Source: CAD feature listing. Evaluate the final solid. Frame: model axes, mm. A direction names the side the tool comes from. Give positions to 0.01 mm unless a question says otherwise; leave off trailing zeros. Order: outer loops, then holes, each group sorted by start corner. A loop starts at its lowest first (then second) coordinate and runs counter-clockwise, first axis right, second up. Notation, with made-up numbers: M 8,19.5 L 44,19.5 A8 ccw 44,31.5 Z; hole C 70.5,53 d11. An arc over 180 degrees is marked long. Answer in a Markdown table with one row per item. Add a question column.
(1) Section query B-B, the plane y = -1.25. Return loops of the section in (x, z) (3 decimals), plus the area to 3 significant figures.
(2) Mould query, pull axis Z, two halves, no side actions, for faces 1 (the face through (8.676, -5.83, 3.645)), 2 (the face through (8.76, 0.51, 3.57)), 3 (the face through (7.13, 0.7, 8.38)), 4 (the face through (-6.3, 1, -6.3)). Classes: pulls with the +Z half, pulls with the -Z half, needs draft (parallel to the pull), parting line crosses it, or undercut.
(3) Section query C-C, the plane z = 3.5. Count the separate pieces of the cut face and the enclosed holes in it, plus the area to 3 significant figures.
(4) Pin query (flat end, axial travel): P1, Ø6, axis at x = 7, y = -1.5, coming from the +Z side; P2, Ø5, axis at x = -3.5, y = -1.5, coming from the -Z side; P3, Ø8, axis at x = 7.5, y = -2, coming from the +Z side. Return the tip coordinate at first contact, or that it passes through.
(5) Section query A-A, the plane x = 0. Return loops of the section in (y, z).
(6) Set-up query: faces 5 (the face through (7.374, -12.007, 2.994)), 6 (the face through (6.786, 0.493, 6.356)), 7 (the face through (8.2, -11.5, 1.4)). Return all of +Z, -Z, +X, -X, +Y, -Y with unobstructed straight access to the full face (end or side cutting, diameter ignored); none if empty.
(7) Material intervals for line 1 along Y through (x, z) = (3, -8.25); line 2 along X through (y, z) = (-6, 0); line 3 along X through (y, z) = (-11.9, 0), sorted ascending.
from build123d import *

# Parameters (mm, degrees)
EXTRUDE_1_DEPTH     = 1
EXTRUDE_START       = 11.5
EXTRUDE_3_DEPTH     = 11.5
EXTRUDE_START_2     = 1
EXTRUDE_4_DEPTH     = 1
FILLET_1_R          = 1
FILLET_2_R          = 1
CUT_EXTRUDE_1_DEPTH = 1.5
SKETCH2_R           = 0.8000000000000002
CUT_EXTRUDE1_DEPTH  = 10


with BuildPart() as part:
    # 草图1 → 凸台-拉伸1 (new body)
    with BuildSketch(Plane(origin=(0, 0, 0), x_dir=(1, 0, 0), z_dir=(0, 1, 0))):
        with BuildLine():
            Line((11.105707880639235, -1.030263157894738), (8.830971038533972, -7.261995457156121))
            Line((8.830971038533972, -7.261995457156121), (5.755000000000001, -9.96795239755889))
            ThreePointArc((5.755000000000001, -9.96795239755889), (-10.633853419204911, 4.404686306522179), (11.117806260587173, 2.9790072091300246))
            Line((11.117806260587173, 2.9790072091300246), (11.105707880639235, -1.030263157894738))
        make_face()
        with BuildLine():
            Line((8.61, 0), (6.102725069252079, -6.073618915368515))
            ThreePointArc((6.102725069252079, -6.073618915368515), (-7.958535130482882, 3.2853947368421053), (8.61, 0))
        make_face(mode=Mode.SUBTRACT)
    extrude(amount=EXTRUDE_1_DEPTH)

    # 草图2 → 凸台-拉伸3 (add)
    with BuildSketch(Plane(origin=(0, 0, 0), x_dir=(-1, 0, 0), z_dir=(0, -1, 0)).offset(EXTRUDE_START)):
        with BuildLine():
            Line((-11.105707880639235, -1.0302631578947385), (-11.117806260587194, 2.979007209129939))
            ThreePointArc((-11.117806260587194, 2.979007209129939), (10.633853419204895, 4.4046863065222155), (-5.755, -9.967952397558888))
            Line((-5.755, -9.967952397558888), (-8.830971038533972, -7.261995457156121))
            Line((-8.830971038533972, -7.261995457156121), (-11.105707880639235, -1.0302631578947385))
        make_face()
        with BuildLine():
            Line((-7.38872176822761, -6.753287394426469), (-9.999910578514989, -0.44931995471382746))
            ThreePointArc((-9.999910578514989, -0.44931995471382746), (9.248034120437978, 3.8306611579745526), (-7.38872176822761, -6.753287394426469))
        make_face(mode=Mode.SUBTRACT)
    extrude(amount=-EXTRUDE_3_DEPTH)

    # 草图5 → 凸台-拉伸4 (add)
    with BuildSketch(Plane(origin=(0, -11.5, 0), x_dir=(-1, 0, 0), z_dir=(0, -1, 0)).offset(EXTRUDE_START_2)):
        with BuildLine():
            Line((-11.117806260587196, 2.9790072091299398), (-11.105707880639235, -1.0302631578947385))
            Line((-11.105707880639235, -1.0302631578947385), (-8.830971038533972, -7.261995457156121))
            Line((-8.830971038533972, -7.261995457156121), (-5.75500000000001, -9.967952397558882))
            ThreePointArc((-5.75500000000001, -9.967952397558882), (10.633853419204897, 4.4046863065222155), (-11.117806260587196, 2.9790072091299398))
        make_face()
        with BuildLine():
            Line((-8.609999999999998, 4.3e-16), (-6.102725069252077, -6.073618915368515))
            ThreePointArc((-6.102725069252077, -6.073618915368515), (7.958535130482882, 3.2853947368421044), (-8.609999999999998, 4.3e-16))
        make_face(mode=Mode.SUBTRACT)
    extrude(amount=-EXTRUDE_4_DEPTH)

    # 圆角1
    # the kernel refuses this fillet: 1 mm, written as the material it takes off along each edge
    with BuildSketch(Plane(origin=(10.708026446892594, -12.5, 5.610734425716317), x_dir=(-0.6605044125759215, 0, -0.7508221633434492), z_dir=(-0.7508221633434492, 0, 0.6605044125759215))) as fillet_1_piece_1:
        with BuildLine():
            CenterArc((FILLET_1_R, -FILLET_1_R), FILLET_1_R, 90, 90)
            Line((-5.1e-16, -FILLET_1_R), (0, 0))
            Line((0, 0), (FILLET_1_R, 0))
        make_face()
    extrude(amount=9.096803728910329, mode=Mode.SUBTRACT)
    with BuildSketch(Plane(origin=(6.9e-16, -12.5, -2.44e-15), x_dir=(0.6755263906448474, 0, 0.7373358092093079), z_dir=(0.7373358092093079, 0, -0.6755263906448474))) as fillet_1_piece_2:
        with BuildLine():
            CenterArc((11.509999999999996 - FILLET_1_R, -FILLET_1_R), FILLET_1_R, 0, 90)
            Line((11.509999999999996 - FILLET_1_R, 0), (11.509999999999996, 0))
            Line((11.509999999999996, 0), (11.509999999999996, -FILLET_1_R))
        make_face()
    revolve(axis=Axis((6.9e-16, -12.5, -2.44e-15), (0, -1, 0)), revolution_arc=309.9900816208065, mode=Mode.SUBTRACT)
    with BuildSketch(Plane(origin=(11.1253502297869, -12.5, -5.47899582680977), x_dir=(0, 1, 0), z_dir=(-0.0030175876798964035, 0, 0.9999954470719326))) as fillet_1_piece_3:
        with BuildLine():
            CenterArc((FILLET_1_R, FILLET_1_R), FILLET_1_R, 180, 90)
            Line((0, FILLET_1_R), (0, 0))
            Line((0, 0), (FILLET_1_R, 0))
        make_face()
    extrude(amount=9.009288621027371, mode=Mode.SUBTRACT)
    with BuildSketch(Plane(origin=(11.962944744412491, -12.5, -1.3181714184535556), x_dir=(7e-17, 1, 3e-17), z_dir=(-0.34289474550930243, 0, 0.9393738305393177))) as fillet_1_piece_4:
        with BuildLine():
            CenterArc((FILLET_1_R, FILLET_1_R), FILLET_1_R, 180, 90)
            Line((-8e-17, FILLET_1_R), (0, 0))
            Line((0, 0), (FILLET_1_R, 0))
        make_face()
    extrude(amount=11.633921551427072, mode=Mode.SUBTRACT)

    # 圆角2
    # the kernel refuses this fillet: 1 mm, written as the material it takes off along each edge
    with BuildSketch(Plane(origin=(11.1253502297869, 1, -5.4789958268098555), x_dir=(0, -1, 0), z_dir=(-0.0030175876798905804, 0, 0.9999954470719326))) as fillet_2_piece_1:
        with BuildLine():
            CenterArc((FILLET_2_R, -FILLET_2_R), FILLET_2_R, 90, 90)
            Line((0, -FILLET_2_R), (0, 0))
            Line((0, 0), (FILLET_2_R, 0))
        make_face()
    extrude(amount=9.009288621027455, mode=Mode.SUBTRACT)
    with BuildSketch(Plane(origin=(9.9e-16, 1, -2.2e-16), x_dir=(0.6755263906448468, 0, 0.7373358092093085), z_dir=(0.7373358092093085, 0, -0.6755263906448468))) as fillet_2_piece_2:
        with BuildLine():
            CenterArc((11.51 - FILLET_2_R, FILLET_2_R), FILLET_2_R, 270, 90)
            Line((11.51 - FILLET_2_R, 0), (11.51, 0))
            Line((11.51, 0), (11.51, FILLET_2_R))
        make_face()
    revolve(axis=Axis((9.9e-16, 1, -2.2e-16), (0, -1, 0)), revolution_arc=309.99008162080594, mode=Mode.SUBTRACT)
    with BuildSketch(Plane(origin=(10.708026446892594, 1, 5.610734425716318), x_dir=(-0.6605044125759214, 0, -0.7508221633434493), z_dir=(-0.7508221633434492, 0, 0.6605044125759213))) as fillet_2_piece_3:
        with BuildLine():
            CenterArc((FILLET_2_R, FILLET_2_R), FILLET_2_R, 180, 90)
            Line((0, FILLET_2_R), (0, 0))
            Line((0, 0), (FILLET_2_R, 0))
        make_face()
    extrude(amount=9.096803728910338, mode=Mode.SUBTRACT)
    with BuildSketch(Plane(origin=(11.962944744412493, 1, -1.318171418453556), x_dir=(-0.9393738305393178, 0, -0.3428947455093024), z_dir=(-0.3428947455093024, 0, 0.9393738305393177))) as fillet_2_piece_4:
        with BuildLine():
            CenterArc((FILLET_2_R, FILLET_2_R), FILLET_2_R, 180, 90)
            Line((-6.1e-16, FILLET_2_R), (0, 0))
            Line((0, 0), (FILLET_2_R, 0))
        make_face()
    extrude(amount=11.633921551427074, mode=Mode.SUBTRACT)

    # 草图7 → 切除-拉伸1 (cut)
    with BuildSketch(Plane(origin=(7.3563625346260375, 0, 3.036809457684256), x_dir=(-0.3815789473684208, 0, 0.9243362520886044), z_dir=(-0.9243362520886044, 0, -0.3815789473684208))):
        Polygon((-3.2853947368421035, 0), (3.2853947368421053, 0), (3.2853947368421057, 1), (-3.2853947368421035, 1), align=None)
    extrude(amount=-CUT_EXTRUDE_1_DEPTH, mode=Mode.SUBTRACT)

    # Sketch2 → Cut-Extrude1 (cut)
    with BuildSketch(Plane(origin=(-10.79858227646779, 0, 3.9838073269619487), x_dir=(0.3461170570774934, 0, 0.938191335922484), z_dir=(-0.938191335922484, 0, 0.34611705707749346))):
        with Locations((0, -5.75)):
            Circle(SKETCH2_R)
    extrude(amount=-CUT_EXTRUDE1_DEPTH, mode=Mode.SUBTRACT)


solid = part.part
Values follow:
| question | item | result |
|---|---|---|
| 1 | outline | M 5.755,9.968 A11.51 ccw long 11.118,-2.979 L 11.106,1.03 L 8.831,7.262 Z; hole M 7.389,6.753 A10.01 ccw long 10,0.449 Z |
| 1 | area | 98.6 mm² |
| 2 | face 1 | undercut |
| 2 | face 2 | undercut |
| 2 | face 3 | pulls with the +Z half |
| 2 | face 4 | needs draft |
| 3 | separate pieces | 3 |
| 3 | enclosed holes | 0 |
| 3 | area | 42.5 mm² |
| 4 | P1 | stops at z = 10.79 |
| 4 | P2 | stops at z = -11.47 |
| 4 | P3 | stops at z = 10.96 |
| 5 | outline | M -12.5,-10.51 A1 ccw -11.5,-11.51 L 0,-11.51 A1 ccw 1,-10.51 L 1,-8.61 L 0,-8.61 L 0,-10.01 L -11.5,-10.01 L -11.5,-8.61 L -12.5,-8.61 Z; M -12.5,8.61 L -11.5,8.61 L -11.5,10.01 L 0,10.01 L 0,8.61 L 1,8.61 L 1,10.51 A1 ccw 0,11.51 L -11.5,11.51 A1 ccw -12.5,10.51 Z |
| 6 | face 5 | +Y, -Y |
| 6 | face 6 | +Y |
| 6 | face 7 | none |
| 7 | line 1 | y = -12.5 to -11.5, 0 to 1 |
| 7 | line 2 | x = -11.51 to -10.01, 10.01 to 11.11 |
| 7 | line 3 | x = -11.43 to -8.61, 8.61 to 11.03 |
